The listing builds one solid part. Answer for the finished solid, in the listing's coordinates (mm). A direction names the side the tool comes from. Coordinates: 2 decimals unless noted, no trailing zeros. Write each loop counter-clockwise with the first axis right and the second up, starting at its lowest first coordinate (ties: lowest second). Pieces come first, ordered by that corner, then holes.
Autodesk Inventor part; units mm, degrees
ref_plane "YZ Plane" through (0, 0, 0) normal (1, 0, 0) x (0, 1, 0)
ref_plane "XZ Plane" through (0, 0, 0) normal (0, 1, 0) x (-1, 0, 0)
ref_plane "XY Plane" through (0, 0, 0) normal (0, 0, 1) x (1, 0, 0)
sketch "Skizze1" plane through (0, 0, 0) normal (0, 0, 1) x (1, 0, 0)
  line L0 (42.6168, 71.3457) -> (-42.6168, 71.3457)
  line L1 (-42.6168, 71.3457) -> (-42.6168, -71.3457)
  line L2 (42.6168, -71.3457) -> (42.6168, 71.3457)
  line L3 (-42.6168, -71.3457) -> (42.6168, -71.3457)
  line L4 (-18, -68.3457) -> (28.5457, -68.3457)
  line L5 (28.5457, -68.3457) -> (39.6168, -57.2746)
  line L6 (39.6168, -57.2746) -> (39.6168, -8.6569)
  line L7 (39.6168, 8.6569) -> (39.6168, 55.2746)
  line L8 (39.6168, 55.2746) -> (26.5457, 68.3457)
  line L9 (26.5457, 68.3457) -> (-26.5457, 68.3457)
  line L10 (-26.5457, 68.3457) -> (-39.6168, 55.2746)
  line L11 (-39.6168, 55.2746) -> (-39.6168, 8.6569)
  line L12 (-39.6168, 8.6569) -> (-30.9599, 0)
  line L13 (-30.9599, 0) -> (-39.6168, -8.6569)
  line L14 (-39.6168, -8.6569) -> (-39.6168, -55.103)
  line L15 (-39.6168, -55.103) -> (-26.3742, -68.3457)
  line L16 (-26.3742, -68.3457) -> (-18, -68.3457)
  line L17 (-42.6168, -56.3457) -> (-27.6168, -71.3457)
  circle A0 centre (37.6168, -66.3457) radius 2.5 construction
  circle A1 centre (36.6168, 0) radius 2.5 construction
  circle A2 centre (-36.6168, 0) radius 2.5 construction
  circle A3 centre (37.6168, -66.3457) radius 2.5 construction
  circle A4 centre (36.6168, 65.3457) radius 2.5 construction
  circle A5 centre (-36.6168, 65.3457) radius 2.5 construction
  line L18 (39.6168, -8.6569) -> (30.9599, 0)
  line L19 (30.9599, 0) -> (39.6168, 8.6569)
  point P0 (0, 0)
  dimension "d0" = 3
  dimension "d1" = 3
  dimension "d2" = 3
  dimension "d3" = 3
  dimension "d4" = 5
  dimension "d5" = 45
  dimension "d6" = 5
  dimension "d7" = 45
  dimension "d8" = 4
  dimension "d9" = 4
  dimension "d10" = 4
  dimension "d11" = 4
  dimension "d12" = 5
  dimension "d13" = 3
  dimension "d14" = 15
extrude "Extrusion1" add sketch "Skizze1" along normal blind 2.5 contours L2 L3 L17 L1 L0
sketch "Skizze2" plane through (0, 0, 0) normal (0, 0, -1) x (-1, 0, 0)
  circle A0 centre (-36.6168, 65.3457) radius 2.4
  circle A1 centre (36.6168, 65.3457) radius 2.4
  circle A2 centre (36.6168, 0) radius 2.4
  circle A3 centre (-36.6168, 0) radius 2.4
  circle A4 centre (-37.6168, -66.3457) radius 2.4
  point P0 (0, 0)
extrude "Extrusion2" add sketch "Skizze2" along normal blind 2.5
sketch "Skizze3" plane through (0, 0, 0) normal (0, 0, -1) x (-1, 0, 0)
  line L0 (42.6168, 71.3457) -> (42.6168, -56.3457)
  line L1 (39.6168, -8.6569) -> (39.6168, -55.103)
  line L2 (42.6168, -40.103) -> (39.6168, -40.103)
  line L3 (39.6168, -40.103) -> (39.6168, -30.103)
  line L4 (39.6168, -30.103) -> (42.6168, -30.103)
  line L5 (42.6168, -30.103) -> (42.6168, -40.103)
  line L6 (-39.6168, -57.2746) -> (-39.6168, -8.6569)
  line L7 (-42.6168, -71.3457) -> (-42.6168, 71.3457)
  line L8 (-39.6168, -40.103) -> (-42.6168, -40.103)
  line L9 (-42.6168, -40.103) -> (-42.6168, -30.103)
  line L10 (-42.6168, -30.103) -> (-39.6168, -30.103)
  line L11 (-39.6168, -30.103) -> (-39.6168, -40.103)
  line L12 (39.6168, -55.103) -> (26.3742, -68.3457)
  line L13 (29.7173, -65.0025) -> (36.7884, -57.9315)
  line L14 (26.3742, -68.3457) -> (39.6168, -55.103)
  line L15 (36.7884, -57.9315) -> (38.9097, -60.0528)
  line L16 (42.6168, -56.3457) -> (27.6168, -71.3457)
  line L17 (38.9097, -60.0528) -> (31.8386, -67.1239)
  line L18 (29.7173, -65.0025) -> (31.8386, -67.1239)
  point P0 (0, 0)
  dimension "d19" = 10
  dimension "d20" = 15
  dimension "d21" = 10
  dimension "d22" = 4
extrude "Extrusion3" cut sketch "Skizze3" against normal blind 1.5 contours L0 L2 L1 L4 | L16 L18 L12 L15 | L8 L7 L10 L6
equation "\"d1\" = d0"
equation "\"d2\" = d0"
equation "\"d3\" = d0"
properties part number "Backplate"
Q1. The part is cut by section A-A, the plane x = 22.5. Write down the section's boundary in (y, z).
Answers below:
outline: (-71.35, 0) - (-68.35, 0) - (-68.35, 2.5) - (-71.35, 2.5) - close; (68.35, 0) - (71.35, 0) - (71.35, 2.5) - (68.35, 2.5) - close
Q2. The part is cut by section B-B, the plane y = 33.5. Write down the section's boundary in (x, z), then the cut area to 3 significant figures.
Answers below:
outline: (-42.62, 0) - (-39.62, 0) - (-39.62, 2.5) - (-42.62, 2.5) - close; (39.62, 0) - (42.62, 0) - (42.62, 2.5) - (39.62, 2.5) - close
area: 15.0 mm2
Q3. Given pin 1 (10 mm diameter, centred on x = -35.5, y = -64.5, fed in from -Z); pin 2 (1.2 mm diameter, centred on x = -41.5, z = 1, fed in from -Y); pin 3 (2.5 mm diameter, centred on x = -41, y = -33.5, fed in from -Z), each flat-ended and moving along its own axis, determine where each tip first touches the part or whether it passes through.
Answers below:
pin 1: stops at z = 0
pin 2: stops at y = -58.06
pin 3: stops at z = 1.5
Q4. Determine the mould class of faces 1 (the face through (-42.617, 8, 1)), 2 (the face through (-35.22, -63.74, 1.79)), 3 (the face through (39.617, 32, 1)) for opening direction Y: released by +Y, released by -Y, zero draft, split by the parting line, or undercut.
Answers below:
face 1: zero draft
face 2: released by -Y
face 3: undercut
Q5. Which of the six approach directions +Z, -Z, +X, -X, +Y, -Y give full straight-line access (tool end or side, diameter ignored) to faces 4 (the face through (-37, 65, -2.5)), 5 (the face through (-41, -35, 1.5)), 6 (the face through (1, 71.346, 1)), 7 (the face through (-35.23, -4.27, 1.23)), 8 (the face through (34.328, -0.721, -1.232))?
Answers below:
face 4: -Z, +X, -X, +Y, -Y
face 5: -Z, +X, -X
face 6: +Z, -Z, +X, -X, +Y
face 7: +Z, -Z
face 8: -Z
Q6. Find the intervals of material crossed by probe 1 along X at (y, z) = (-43, 1.15); probe 2 along Y at (x, z) = (34.5, 0.9); probe 3 along Y at (x, z) = (14.5, 2), in increasing order.
Answers below:
probe 1: x = -42.62 to -39.62, 39.62 to 42.62
probe 2: y = -71.35 to -62.39, -3.54 to 3.54, 60.39 to 71.35
probe 3: y = -71.35 to -68.35, 68.35 to 71.35
